Check sheet for the modelled part. Datum: model origin and axes. Units: mm. A direction names the side the tool comes from. Round coordinates to 2 decimals unless told otherwise and drop trailing zeros. Order: outer loops, then holes, each group sorted by start corner. A loop starts at its lowest first (then second) coordinate and runs counter-clockwise, first axis right, second up. Notation, with made-up numbers: (18, -39) -> (72, -39) arc R10 ccw to (72, -28) -> close; hole circle Ø5 at (-4.5, 88.25). An arc over 180 degrees is marked (long way). Answer in a Markdown table with one row per item.
```python
from build123d import *

# Parameters (mm, degrees)
SKETCH1_W           = 10.16
SKETCH1_H           = 6.35
BOSS_EXTRUDE1_DEPTH = 2.286
SKETCH2_W           = 5.842
SKETCH2_H           = 1.778
CUT_EXTRUDE1_DEPTH  = 8.89
SKETCH3_W           = 5.08
SKETCH3_H           = 6.35
BOSS_EXTRUDE2_DEPTH = 5.08
SKETCH4_W           = 20.32
SKETCH4_H           = 3.4036
BOSS_EXTRUDE3_DEPTH = 32.004


with BuildPart() as part:
    # Sketch1 → Boss-Extrude1 (new body)
    with BuildSketch(Plane(origin=(0, 0, 0), x_dir=(1, 0, 0), z_dir=(0, 1, 0))):
        with Locations((5.08, 3.175)):
            Rectangle(SKETCH1_W, SKETCH1_H)
    extrude(amount=BOSS_EXTRUDE1_DEPTH)

    # Sketch2 → Cut-Extrude1 (cut)
    with BuildSketch(Plane.ZY):
        with Locations((-3.1242, 1.0922)):
            Rectangle(SKETCH2_W, SKETCH2_H)
    extrude(amount=-CUT_EXTRUDE1_DEPTH, mode=Mode.SUBTRACT)

    # Sketch3 → Boss-Extrude2 (add)
    with BuildSketch(Plane.XZ):
        with Locations((7.62, -3.175)):
            Rectangle(SKETCH3_W, SKETCH3_H)
    extrude(amount=BOSS_EXTRUDE2_DEPTH)

    # Sketch4 → Boss-Extrude3 (add)
    with BuildSketch(Plane(origin=(10.16, 0, 0), x_dir=(0, 0, -1), z_dir=(1, 0, 0))):
        with Locations((3.175, -3.3782)):
            Rectangle(SKETCH4_W, SKETCH4_H)
    extrude(amount=BOSS_EXTRUDE3_DEPTH)


solid = part.part
```
(1) Draft check along Z on faces 5 (the flat face through (26, -3, 6.985)), 6 (the flat face through (10.16, -3, -10)), 7 (the flat face through (4, 1, -6.045)). Enter one of: pulls with the +Z half, pulls with the -Z half, needs draft (parallel to the pull), parting line crosses it, or undercut.
Solutions:
| item | result |
|---|---|
| face 5 | pulls with the +Z half |
| face 6 | needs draft |
| face 7 | undercut |
(2) Scan lines: probe 1 along Z at (x, y) = (6.5, 0.5); probe 2 along Y at (x, z) = (5, -6); probe 3 along Y at (x, z) = (34, -11.5). Record each from-to range of solid material in increasing order. Write a range as from..to.
Solutions:
| item | result |
|---|---|
| probe 1 | -6.35..-6.05, -0.2..0 |
| probe 2 | 0..0.2, 1.98..2.29 |
| probe 3 | -5.08..-1.68 |
(3) Depth check by flat-ended pin: pin 1 Ø10 at (x, z) = (26, 0.5) entering from +Y; pin 2 Ø1.7 at (y, z) = (-3.5, 2.5) entering from -X; pin 3 Ø2 at (x, y) = (11, -0.5) entering from -Z. Enter the tip coordinate at first touch or a pass-through.
Solutions:
| item | result |
|---|---|
| pin 1 | y = -1.68 |
| pin 2 | x = 10.16 |
| pin 3 | z = -6.35 |
(4) Section check D-D on x = 23.5. Record the boundary of the cut face in (y, z) (3 decimals), plus the area to 3 significant figures.
Solutions:
| item | result |
|---|---|
| outline | (-5.08, -13.335) -> (-1.676, -13.335) -> (-1.676, 6.985) -> (-5.08, 6.985) -> close |
| area | 69.2 mm^2 |
(5) Section check B-B on y = -2.25. Record the boundary of the cut face in (x, z) (3 decimals), plus the area to 3 significant figures.
Solutions:
| item | result |
|---|---|
| outline | (5.08, -6.35) -> (10.16, -6.35) -> (10.16, -13.335) -> (42.164, -13.335) -> (42.164, 6.985) -> (10.16, 6.985) -> (10.16, 0) -> (5.08, 0) -> close |
| area | 683 mm^2 |
(6) Section check A-A on z = -3.25. Record the boundary of the cut face in (x, y).
Solutions:
| item | result |
|---|---|
| outline | (0, 0) -> (5.08, 0) -> (5.08, -5.08) -> (42.16, -5.08) -> (42.16, -1.68) -> (10.16, -1.68) -> (10.16, 2.29) -> (0, 2.29) -> (0, 1.98) -> (8.89, 1.98) -> (8.89, 0.2) -> (0, 0.2) -> close |
(7) Section check C-C on y = 1. Record the boundary of the cut face in (x, z).
Solutions:
| item | result |
|---|---|
| outline | (0, -6.35) -> (10.16, -6.35) -> (10.16, 0) -> (0, 0) -> (0, -0.2) -> (8.89, -0.2) -> (8.89, -6.05) -> (0, -6.05) -> close |
(8) Tool access check on faces 1 (the flat face through (5.08, -3, -3)), 2 (the flat face through (10.16, 0, -3)), 3 (the flat face through (8.89, 1, -3)), 4 (the flat face through (6, -1, -6.35)). Record the directions out of +Z, -Z, +X, -X, +Y, -Y that give a thin tool (end or side, any length) a straight path to the whole face; none if there is none.
Solutions:
| item | result |
|---|---|
| face 1 | +Z, -Z, -X, -Y |
| face 2 | +Z, -Z, +X, +Y |
| face 3 | -X |
| face 4 | -Z, -X, +Y, -Y |
